Here's how the part is built. I have some questions about the finished solid (model axes, mm). A direction names the side the tool comes from. Coordinates: 2 decimals unless noted, no trailing zeros. Write each loop counter-clockwise with the first axis right and the second up, starting at its lowest first coordinate (ties: lowest second). Pieces come first, ordered by that corner, then holes. Notation, with made-up numbers: M -18,8.5 L -6,8.5 A12 cw -6,22.5 Z; hole C 34.25,83.25 d9. An arc over 180 degrees is marked long. Use a Markdown table: item, result.
```python
from build123d import *

# Parameters (mm, degrees)
BOSS_EXTRU_1_DEPTH      = 6
ENL_V_MAT_EXTRU_2_DEPTH = 6
CHANFREIN1_SIZE         = 3
ESQUISSE4_R             = 1.8
ESQUISSE4_W             = 7
ESQUISSE4_H             = 9.3
ENL_V_MAT_EXTRU_3_DEPTH = 6
CHANFREIN2_SIZE         = 7
BOSS_EXTRU_2_DEPTH      = 6
ESQUISSE11_R            = 2
ENL_V_MAT_EXTRU_6_DEPTH = 6
ESQUISSE12_R            = 1.5
ENL_V_MAT_EXTRU_7_DEPTH = 10


with BuildPart() as part:
    # Esquisse1 → Boss.-Extru.1 (new body)
    with BuildSketch(Plane(origin=(0, 0, 0), x_dir=(1, 0, 0), z_dir=(0, 1, 0))):
        Polygon((0, 0), (0, 110), (-8, 110), (-28, 90), (-78, 90), (-98, 110), (-110, 110), (-110, 98), (-75, 63), (-75, 41), (-110, 6), (-110, 0), align=None)
    extrude(amount=BOSS_EXTRU_1_DEPTH)

    # Esquisse3 → Enlèv. mat.-Extru.2 (cut)
    with BuildSketch(Plane(origin=(0, 0, 0), x_dir=(1, 0, 0), z_dir=(0, 1, 0))):
        Polygon((0, 70), (-58, 70), (-23, 35), (0, 35), align=None)
    extrude(amount=ENL_V_MAT_EXTRU_2_DEPTH, mode=Mode.SUBTRACT)

    # Chanfrein1
    chanfrein1_edges = [part.edges().sort_by_distance(p)[0] for p in [
        (-110, 3, -110),
    ]]
    chamfer(chanfrein1_edges, length=CHANFREIN1_SIZE)

    # Symétrie3: part across plane


with BuildPart() as part_1:
    add(part.part)
    add(part.part.mirror(Plane(origin=(-110, 6, 0), x_dir=(1, 0, 0), z_dir=(0, 0, -1))))

    # Esquisse4 → Enlèv. mat.-Extru.3 (cut)
    with BuildSketch(Plane(origin=(0, 6, 0), x_dir=(1, 0, 0), z_dir=(0, 1, 0))):
        with Locations((-7.5, 0)):
            Circle(ESQUISSE4_R)
        Polygon((-45, 30.405591591), (-14.594408409, 0), (-45, -30.405591591), (-75.405591591, 0), align=None)
        with Locations((-7.5, 11.65)):
            Rectangle(ESQUISSE4_W, ESQUISSE4_H)
        with Locations((-7.5, -11.65)):
            Rectangle(ESQUISSE4_W, ESQUISSE4_H)
    extrude(amount=-ENL_V_MAT_EXTRU_3_DEPTH, mode=Mode.SUBTRACT)

    # Chanfrein2
    chanfrein2_edges = [part_1.edges().sort_by_distance(p)[0] for p in [
        (-14.594408409, 3, 0),
        (-45, 3, 30.405591591),
        (-75.405591591, 3, 0),
        (-45, 3, -30.405591591),
    ]]
    chamfer(chanfrein2_edges, length=CHANFREIN2_SIZE)

    # Symétrie5: part across plane


with BuildPart() as part_2:
    add(part_1.part)
    add(part_1.part.mirror(Plane(origin=(0, 6, 0), x_dir=(0, 0, 1), z_dir=(-1, 0, 0))))

    # Esquisse8 → Boss.-Extru.2 (add)
    with BuildSketch(Plane(origin=(0, 6, 0), x_dir=(1, 0, 0), z_dir=(0, 1, 0))):
        Polygon((100, 16), (100, 53), (90, 63), (90, 78), (75, 63), (75, 41), align=None)
    boss_extru_2 = extrude(amount=-BOSS_EXTRU_2_DEPTH)

    # Esquisse11 → Enlèv. mat.-Extru.6 (cut)
    with BuildSketch(Plane(origin=(0, 6, 0), x_dir=(1, 0, 0), z_dir=(0, 1, 0))):
        with Locations((-105, 105)):
            Circle(ESQUISSE11_R)
        with Locations((0, 105)):
            Circle(ESQUISSE11_R)
        with Locations((105, 105)):
            Circle(ESQUISSE11_R)
        with Locations((105, 0)):
            Circle(ESQUISSE11_R)
        with Locations((105, -105)):
            Circle(ESQUISSE11_R)
        with Locations((0, -105)):
            Circle(ESQUISSE11_R)
        with Locations((-105, -105)):
            Circle(ESQUISSE11_R)
        with Locations((-105, 0)):
            Circle(ESQUISSE11_R)
    extrude(amount=-ENL_V_MAT_EXTRU_6_DEPTH, mode=Mode.SUBTRACT)

    # Symétrie6: Boss.-Extru.2 across plane
    add(boss_extru_2.mirror(Plane.XY))

    # Esquisse12 → Enlèv. mat.-Extru.7 (cut)
    with BuildSketch(Plane(origin=(0, 6, 0), x_dir=(1, 0, 0), z_dir=(0, 1, 0))):
        with Locations((-94.75, 0)):
            Circle(ESQUISSE12_R)
        with Locations((-75.25, 0)):
            Circle(ESQUISSE12_R)
        with Locations((75.25, 35)):
            Circle(ESQUISSE12_R)
        with Locations((94.75, 35)):
            Circle(ESQUISSE12_R)
        with Locations((75.25, -35)):
            Circle(ESQUISSE12_R)
        with Locations((94.75, -35)):
            Circle(ESQUISSE12_R)
        with BuildLine():
            Line((-86, 15.5), (-84, 15.5))
            ThreePointArc((-84, 15.5), (-81.171572875, 14.328427125), (-80, 11.5))
            Line((-80, 11.5), (-80, -11.5))
            ThreePointArc((-80, -11.5), (-81.171572875, -14.328427125), (-84, -15.5))
            Line((-84, -15.5), (-86, -15.5))
            ThreePointArc((-86, -15.5), (-88.828427125, -14.328427125), (-90, -11.5))
            Line((-90, -11.5), (-90, 11.5))
            ThreePointArc((-90, 11.5), (-88.828427125, 14.328427125), (-86, 15.5))
        make_face()
        with BuildLine():
            Line((84, 50.5), (86, 50.5))
            ThreePointArc((86, 50.5), (88.828427125, 49.328427125), (90, 46.5))
            Line((90, 46.5), (90, 23.5))
            ThreePointArc((90, 23.5), (88.828427125, 20.671572875), (86, 19.5))
            Line((86, 19.5), (84, 19.5))
            ThreePointArc((84, 19.5), (81.171572875, 20.671572875), (80, 23.5))
            Line((80, 23.5), (80, 46.5))
            ThreePointArc((80, 46.5), (81.171572875, 49.328427125), (84, 50.5))
        make_face()
        with BuildLine():
            Line((84, -19.5), (86, -19.5))
            ThreePointArc((86, -19.5), (88.828427125, -20.671572875), (90, -23.5))
            Line((90, -23.5), (90, -46.5))
            ThreePointArc((90, -46.5), (88.828427125, -49.328427125), (86, -50.5))
            Line((86, -50.5), (84, -50.5))
            ThreePointArc((84, -50.5), (81.171572875, -49.328427125), (80, -46.5))
            Line((80, -46.5), (80, -23.5))
            ThreePointArc((80, -23.5), (81.171572875, -20.671572875), (84, -19.5))
        make_face()
    extrude(amount=-ENL_V_MAT_EXTRU_7_DEPTH, mode=Mode.SUBTRACT)


solid = part_2.part
```
1. I need wall thicknesses on probe 1 along Z at (x, y) = (0, 3.6); probe 2 along Z at (x, y) = (7.5, 3.15); probe 3 along Z at (x, y) = (-2.5, 1.85). Which ranges of each line are inside material? Lowest first, please.
Answers follow:
| item | result |
|---|---|
| probe 1 | z = -110 to -107, -103 to -70, -35 to 35, 70 to 103, 107 to 110 |
| probe 2 | z = -110 to -70, -35 to -16.3, -7 to -1.8, 1.8 to 7, 16.3 to 35, 70 to 110 |
| probe 3 | z = -110 to -70, -35 to 35, 70 to 110 |
2. Suppose I cut it at B-B on y = 4.6. State how many separate pieces and enclosed holes the cut face has, and give its area (3 significant figures).
Answers follow:
| item | result |
|---|---|
| separate pieces | 1 |
| enclosed holes | 27 |
| area | 26,200 mm2 |
3. Suppose I cut it at C-C on z = -72.5. Write out the boundary of the cut face in (x, y).
Answers follow:
| item | result |
|---|---|
| outline | M -84.5,0 L 90,0 L 90,6 L -84.5,6 Z |
4. Which directions (+Z, -Z, +X, -X, +Y, -Y) give clear straight access to the entire face, cutting with the end or side of a thin tool? Please do faces 1 (the face through (-110, 3, -103)), 2 (the face through (0, 3, 110)), 3 (the face through (-8, 3, -7)), 4 (the face through (-88, 3, 100)), 5 (the face through (100, 3, 34)).
Answers follow:
| item | result |
|---|---|
| face 1 | +Z, -Z, -X, +Y, -Y |
| face 2 | +Z, +X, -X, +Y, -Y |
| face 3 | +Y, -Y |
| face 4 | +Z, +Y, -Y |
| face 5 | +X, +Y, -Y |
5. Suppose I cut it at A-A on x = 54.5. Write out the boundary of the cut face in (y, z).
Answers follow:
| item | result |
|---|---|
| outline | M 0,-90 L 6,-90 L 6,-70 L 0,-70 Z; M 0,-66.5 L 6,-66.5 L 6,-20.91 L 0,-20.91 Z; M 0,20.91 L 6,20.91 L 6,66.5 L 0,66.5 Z; M 0,70 L 6,70 L 6,90 L 0,90 Z |
6. Will these pins go through, and if not, where does the flat tip stop? pin 1 Ø1.5 at (x, y) = (37, 0.5) entering from +Z; pin 2 Ø1.8 at (y, z) = (2, -39.5) entering from +X; pin 3 Ø3 at (x, z) = (0, -105) entering from +Y; pin 4 Ø2 at (x, y) = (17, 3.5) entering from +Z.
Answers follow:
| item | result |
|---|---|
| pin 1 | stops at z = 90 |
| pin 2 | stops at x = 100 |
| pin 3 | passes through |
| pin 4 | stops at z = 102 |
7. We'd pull the mould along Z, two halves only. Please class faces 6 (the face through (11, 3, 12)), 7 (the face through (-8, 3, 7)), 8 (the face through (18, 3, 100)), 9 (the face through (110, 3, 0)): +Z half, -Z half, draft (parallel to the pull), parting line (faces both ways), or undercut.
Answers follow:
| item | result |
|---|---|
| face 6 | undercut |
| face 7 | undercut |
| face 8 | +Z half |
| face 9 | draft |
